CAD build for the part. Positions are in the model's coordinates, mm. Give positions to 0.01 mm unless a question says otherwise; leave off trailing zeros. Order: outer loops, then holes, each group sorted by start corner. A loop starts at its lowest first (then second) coordinate and runs counter-clockwise, first axis right, second up.
from build123d import *

# Parameters (mm, degrees)
SKETCH1_R           = 30
BOSS_EXTRUDE1_DEPTH = 2
CUT_EXTRUDE3_REACH  = 44.474
SKETCH4_R           = 11
SKETCH4_R_2         = 1.5
SKETCH4_R_3         = 2


with BuildPart() as part:
    # Sketch1 → Boss-Extrude1 (new body)
    with BuildSketch(Plane(origin=(0, 0, 0), x_dir=(1, 0, 0), z_dir=(0, 1, 0))):
        with Locations(Location((0, 0, 0), (0, 0, 270))):
            Circle(SKETCH1_R)
    extrude(amount=BOSS_EXTRUDE1_DEPTH)

    # Sketch4 → Cut-Extrude3 (cut, up to next)
    with BuildSketch(Plane(origin=(0, 2, 0), x_dir=(1, 0, 0), z_dir=(0, 1, 0)), mode=Mode.PRIVATE) as cut_extrude3_sk1:
        with Locations(Location((-4.949747468, 4.949747468, 0), (0, 0, 270))):
            Circle(SKETCH4_R)
    cut_extrude3_tool1 = extrude(cut_extrude3_sk1.sketch, amount=-CUT_EXTRUDE3_REACH, mode=Mode.PRIVATE) & part.part
    # Sketch4 → Cut-Extrude3 (cut, up to next)
    with BuildSketch(Plane(origin=(0, 2, 0), x_dir=(1, 0, 0), z_dir=(0, 1, 0)), mode=Mode.PRIVATE) as cut_extrude3_sk2:
        with Locations(Location((-4.949747468, 18.449747468, 0), (0, 0, 270))):
            Circle(SKETCH4_R_2)
    cut_extrude3_tool2 = extrude(cut_extrude3_sk2.sketch, amount=-CUT_EXTRUDE3_REACH, mode=Mode.PRIVATE) & part.part
    # Sketch4 → Cut-Extrude3 (cut, up to next)
    with BuildSketch(Plane(origin=(0, 2, 0), x_dir=(1, 0, 0), z_dir=(0, 1, 0)), mode=Mode.PRIVATE) as cut_extrude3_sk3:
        with Locations(Location((6.741595483, 11.699747468, 0), (0, 0, 270))):
            Circle(SKETCH4_R_2)
    cut_extrude3_tool3 = extrude(cut_extrude3_sk3.sketch, amount=-CUT_EXTRUDE3_REACH, mode=Mode.PRIVATE) & part.part
    # Sketch4 → Cut-Extrude3 (cut, up to next)
    with BuildSketch(Plane(origin=(0, 2, 0), x_dir=(1, 0, 0), z_dir=(0, 1, 0)), mode=Mode.PRIVATE) as cut_extrude3_sk4:
        with Locations(Location((6.741595483, -1.800252532, 0), (0, 0, 270))):
            Circle(SKETCH4_R_2)
    cut_extrude3_tool4 = extrude(cut_extrude3_sk4.sketch, amount=-CUT_EXTRUDE3_REACH, mode=Mode.PRIVATE) & part.part
    # Sketch4 → Cut-Extrude3 (cut, up to next)
    with BuildSketch(Plane(origin=(0, 2, 0), x_dir=(1, 0, 0), z_dir=(0, 1, 0)), mode=Mode.PRIVATE) as cut_extrude3_sk5:
        with Locations(Location((-4.949747468, -8.550252532, 0), (0, 0, 270))):
            Circle(SKETCH4_R_2)
    cut_extrude3_tool5 = extrude(cut_extrude3_sk5.sketch, amount=-CUT_EXTRUDE3_REACH, mode=Mode.PRIVATE) & part.part
    # Sketch4 → Cut-Extrude3 (cut, up to next)
    with BuildSketch(Plane(origin=(0, 2, 0), x_dir=(1, 0, 0), z_dir=(0, 1, 0)), mode=Mode.PRIVATE) as cut_extrude3_sk6:
        with Locations(Location((-16.641090419, -1.800252532, 0), (0, 0, 270))):
            Circle(SKETCH4_R_2)
    cut_extrude3_tool6 = extrude(cut_extrude3_sk6.sketch, amount=-CUT_EXTRUDE3_REACH, mode=Mode.PRIVATE) & part.part
    # Sketch4 → Cut-Extrude3 (cut, up to next)
    with BuildSketch(Plane(origin=(0, 2, 0), x_dir=(1, 0, 0), z_dir=(0, 1, 0)), mode=Mode.PRIVATE) as cut_extrude3_sk7:
        with Locations(Location((-16.641090419, 11.699747468, 0), (0, 0, 270))):
            Circle(SKETCH4_R_2)
    cut_extrude3_tool7 = extrude(cut_extrude3_sk7.sketch, amount=-CUT_EXTRUDE3_REACH, mode=Mode.PRIVATE) & part.part
    # Sketch4 → Cut-Extrude3 (cut, up to next)
    with BuildSketch(Plane(origin=(0, 2, 0), x_dir=(1, 0, 0), z_dir=(0, 1, 0)), mode=Mode.PRIVATE) as cut_extrude3_sk8:
        with Locations(Location((-4.949747468, -17.777677021, 0), (0, 0, 270))):
            Circle(SKETCH4_R_3)
    cut_extrude3_tool8 = extrude(cut_extrude3_sk8.sketch, amount=-CUT_EXTRUDE3_REACH, mode=Mode.PRIVATE) & part.part
    # Sketch4 → Cut-Extrude3 (cut, up to next)
    with BuildSketch(Plane(origin=(0, 2, 0), x_dir=(1, 0, 0), z_dir=(0, 1, 0)), mode=Mode.PRIVATE) as cut_extrude3_sk9:
        with Locations(Location((12.02081528, -12.02081528, 0), (0, 0, 270))):
            Circle(SKETCH4_R_3)
    cut_extrude3_tool9 = extrude(cut_extrude3_sk9.sketch, amount=-CUT_EXTRUDE3_REACH, mode=Mode.PRIVATE) & part.part
    # Sketch4 → Cut-Extrude3 (cut, up to next)
    with BuildSketch(Plane(origin=(0, 2, 0), x_dir=(1, 0, 0), z_dir=(0, 1, 0)), mode=Mode.PRIVATE) as cut_extrude3_sk10:
        with Locations(Location((17.777677021, 4.949747468, 0), (0, 0, 270))):
            Circle(SKETCH4_R_3)
    cut_extrude3_tool10 = extrude(cut_extrude3_sk10.sketch, amount=-CUT_EXTRUDE3_REACH, mode=Mode.PRIVATE) & part.part
    # Sketch4 → Cut-Extrude3 (cut, up to next)
    with BuildSketch(Plane(origin=(0, 2, 0), x_dir=(1, 0, 0), z_dir=(0, 1, 0)), mode=Mode.PRIVATE) as cut_extrude3_sk11:
        with Locations(Location((11.050252532, 18.449747468, 0), (0, 0, 270))):
            Circle(SKETCH4_R_3)
    cut_extrude3_tool11 = extrude(cut_extrude3_sk11.sketch, amount=-CUT_EXTRUDE3_REACH, mode=Mode.PRIVATE) & part.part
    # Sketch4 → Cut-Extrude3 (cut, up to next)
    with BuildSketch(Plane(origin=(0, 2, 0), x_dir=(1, 0, 0), z_dir=(0, 1, 0)), mode=Mode.PRIVATE) as cut_extrude3_sk12:
        with Locations(Location((-16.641090419, -12.02081528, 0), (0, 0, 270))):
            Circle(SKETCH4_R_3)
    cut_extrude3_tool12 = extrude(cut_extrude3_sk12.sketch, amount=-CUT_EXTRUDE3_REACH, mode=Mode.PRIVATE) & part.part
    add(cut_extrude3_tool1.solids().sort_by_distance((-4.949747, 2, -4.949747))[0], mode=Mode.SUBTRACT)
    add(cut_extrude3_tool2.solids().sort_by_distance((-4.949747, 2, -18.449747))[0], mode=Mode.SUBTRACT)
    add(cut_extrude3_tool3.solids().sort_by_distance((6.741595, 2, -11.699747))[0], mode=Mode.SUBTRACT)
    add(cut_extrude3_tool4.solids().sort_by_distance((6.741595, 2, 1.800253))[0], mode=Mode.SUBTRACT)
    add(cut_extrude3_tool5.solids().sort_by_distance((-4.949747, 2, 8.550253))[0], mode=Mode.SUBTRACT)
    add(cut_extrude3_tool6.solids().sort_by_distance((-16.64109, 2, 1.800253))[0], mode=Mode.SUBTRACT)
    add(cut_extrude3_tool7.solids().sort_by_distance((-16.64109, 2, -11.699747))[0], mode=Mode.SUBTRACT)
    add(cut_extrude3_tool8.solids().sort_by_distance((-4.949747, 2, 17.777677))[0], mode=Mode.SUBTRACT)
    add(cut_extrude3_tool9.solids().sort_by_distance((12.020815, 2, 12.020815))[0], mode=Mode.SUBTRACT)
    add(cut_extrude3_tool10.solids().sort_by_distance((17.777677, 2, -4.949747))[0], mode=Mode.SUBTRACT)
    add(cut_extrude3_tool11.solids().sort_by_distance((11.050253, 2, -18.449747))[0], mode=Mode.SUBTRACT)
    add(cut_extrude3_tool12.solids().sort_by_distance((-16.64109, 2, 12.020815))[0], mode=Mode.SUBTRACT)


solid = part.part
1. Pin check, flat tips, straight feed: P1, Ø6.5, axis at x = -4.95, z = 17.78, coming from the +Y side; P2, Ø1, axis at y = 1, z = -7, coming from the -X side; P3, Ø1, axis at y = 1, z = 14, coming from the -X side. Stop position of each tip, or through.
2. Saw through at B-B on z = 19. Give the cut face in (x, y).
3. Wall check: line 1 (Z direction, x = -16.5, y = 1.6); line 2 (X direction, y = 0.1, z = -18); line 3 (X direction, y = 0.75, z = 3). Give the ranges that are in metal, low to high.
4. Saw through at C-C on y = 1.55. State how many separate pieces and enclosed holes the cut face has, plus the area to 3 significant figures.
5. Mould opens along Z. For faces 1 (the cylindrical face through (1.32, 0.99, -29.97)), 2 (the cylindrical face through (15.825, 1.014, -5.383)), 3 (the flat face through (0, 0, 6)) say: released by +Z, released by -Z, zero draft, split by the parting line, or undercut.
6. Saw through at A-A on x = 0. Give the cut face in (y, z), plus the area to 3 significant figures.
7. Saw through at D-D on x = 23. Give the cut face in (y, z), plus the area to 3 significant figures.
Reported:
1. P1: stops at y = 2
1. P2: stops at x = -29.29
1. P3: stops at x = -26.79
2. outline: (-23.22, 0) - (-6.53, 0) - (-6.53, 2) - (-23.22, 2) - close; (-3.37, 0) - (23.22, 0) - (23.22, 2) - (-3.37, 2) - close
3. line 1: z = -25.05 to -13.19, -10.21 to 0.31, 3.29 to 10.03, 14.02 to 25.05
3. line 2: x = -24 to -6.38, -3.52 to 9.1, 13 to 24
3. line 3: x = -29.85 to -17.54, -15.74 to -12.55, 2.65 to 5.84, 7.64 to 29.85
4. separate pieces: 1
4. enclosed holes: 12
4. area: 2,340 mm2
5. face 1: split by the parting line
5. face 2: undercut
5. face 3: zero draft
6. outline: (0, -30) - (2, -30) - (2, -14.77) - (0, -14.77) - close; (0, 4.87) - (2, 4.87) - (2, 30) - (0, 30) - close
6. area: 80.7 mm2
7. outline: (0, -19.26) - (2, -19.26) - (2, 19.26) - (0, 19.26) - close
7. area: 77.0 mm2
